CAD build for the part. Positions are in the model's coordinates, mm. A direction names the side the tool comes from. Give positions to 0.01 mm unless a question says otherwise; leave off trailing zeros. Loops run counter-clockwise (first coordinate to the right, second up) from the corner with the lowest first, then second, coordinate; pieces in that order, holes last. Notation, with made-up numbers: (-39, -13) -> (-33, -13) arc R25 ccw to (-33, 26) -> close; hole circle Ø4 at (-10, 28.5). An arc over 180 degrees is marked (long way). Write each question's results on one line, items separated by ' | '. Start each with the question number.
```python
from build123d import *

# Parameters (mm, degrees)
ESTRUSIONE_ESTRUSIONE1_DEPTH = 12.54
SCHIZZO3_R                   = 6.5
ESTRUSIONE_ESTRUSIONE2_DEPTH = 2.62
SCHIZZO4_R                   = 3
TAGLIO_ESTRUSIONE1_DEPTH     = 36.652428389
FORO_FILETTATO_M2_5X0_45_1_D = 2.05


with BuildPart() as part:
    # Schizzo1 → Rivoluzione1 (revolve)
    with BuildSketch(Plane.XY, mode=Mode.PRIVATE) as rivoluzione1_sk:
        with BuildLine():
            Line((0, 0), (9.485, 0))
            Line((9.485, 0), (9.485, -4.2))
            Line((9.485, -4.2), (14.505, -4.2))
            Line((14.505, -4.2), (14.505, -7.3))
            Line((14.505, -7.3), (10.745, -7.3))
            ThreePointArc((10.745, -7.3), (9.154009742, -7.959009742), (8.495, -9.55))
            Line((8.495, -9.55), (8.495, -14))
            Line((8.495, -14), (0, -14))
            Line((0, -14), (0, 0))
        make_face()
    revolve(rivoluzione1_sk.sketch.rotate(Axis((0, 0, 0), (0, -1, 0)), 180), axis=Axis((0, 0, 0), (0, -1, 0)))

    # Schizzo2 → Estrusione-Estrusione1 (add)
    with BuildSketch(Plane(origin=(0, 0, 0), x_dir=(1, 0, 0), z_dir=(0, 1, 0))):
        Polygon((2.090015263, -8.937889289), (3.249793028, -8.584455371), (8.785446812, -2.658938333), (9.059252943, -1.477824366), (6.695431549, 6.278950956), (5.809459915, 7.106631005), (-2.090015263, 8.937889289), (-3.249793028, 8.584455371), (-8.785446812, 2.658938333), (-9.059252943, 1.477824366), (-6.695431549, -6.278950956), (-5.809459915, -7.106631005), align=None)
    extrude(amount=ESTRUSIONE_ESTRUSIONE1_DEPTH)

    # Schizzo3 → Estrusione-Estrusione2 (add)
    with BuildSketch(Plane(origin=(0, 12.54, 0), x_dir=(1, 0, 0), z_dir=(0, 1, 0))):
        with Locations(Location((0, 0, 0), (0, 0, 180))):
            Circle(SCHIZZO3_R)
    extrude(amount=ESTRUSIONE_ESTRUSIONE2_DEPTH)

    # Schizzo4 → Taglio-Estrusione1 (cut, through all)
    with BuildSketch(Plane(origin=(0, 15.16, 0), x_dir=(1, 0, 0), z_dir=(0, 1, 0))):
        with Locations(Location((0, 0, 0), (0, 0, 180))):
            Circle(SCHIZZO4_R)
    extrude(amount=-TAGLIO_ESTRUSIONE1_DEPTH, mode=Mode.SUBTRACT)

    # Foro filettato M2.5x0.45-1 (through all)
    with Locations(Plane(origin=(0, -4.2, 0), x_dir=(1, 0, 0), z_dir=(0, 1, 0))):
        with Locations((0, -12), (-10.392304845, -6), (-10.392304845, 6), (0, 12), (10.392304845, 6), (10.392304845, -6), (0, 0)):
            Hole(FORO_FILETTATO_M2_5X0_45_1_D / 2)


solid = part.part
```
Q1. Saw through at C-C, the plane z = 0. List the corners of the cut face in (x, y) (3 decimals), then the cut area to 3 significant figures.
Q2. Which spindle directions (+Z, -Z, +X, -X, +Y, -Y) get a long thin tool onto all of the face, cutting with end or side? Do faces 1 (the face through (-6.259, 6.182, 6.687)), 2 (the face through (-8.92, 6.18, -2.08)), 3 (the face through (1.842, -11.806, 8.293)), 4 (the face through (5.158, 13.832, -3.955)), 5 (the face through (1.92, 6.18, -8.01)). Say none if no direction does.
Q3. Wall check: L1, parallel to X at y = -5.1, z = 6; L2, parallel to X at y = -0.75, z = -0.25; L3, parallel to Y at x = 8.5, z = -11.5. Give the ranges that are in metal, low to high.
Q4. Drop flat-ended pins along their axis: pin 1 (2.5 mm diameter, centred on x = -10.39, z = 6, fed in from -Y); pin 2 (2.5 mm diameter, centred on x = -10.39, z = -6, fed in from +Y); pin 3 (1.8 mm diameter, centred on x = 0, z = -12, fed in from -Y); pin 4 (1.5 mm diameter, centred on y = 11, z = 2.5, fed in from -X). Give the stop position or say it passes through.
Q5. Saw through at B-B, the plane y = -4.75. List the corners of the cut face in (x, z) (3 decimals), then the cut area to 3 significant figures.
Q6. Saw through at D-D, the plane x = 0. Give the number of separate pieces and of enclosed holes in the cut face, then the cut area to 3 significant figures.
Q7. Mould opens along X. For faces 6 (the face through (3.14, -5.77, 14.16)), 7 (the face through (0, 12.54, 7)), 8 (the face through (0.76, -5.77, 11.31)), 9 (the face through (8.92, 6.18, 2.08)) say: pulls with the +X half, pulls with the -X half, needs draft (parallel to the pull), parting line crosses it, or undercut.
Q8. Saw through at A-A, the plane y = 8.5. List the corners of the cut face in (x, z), then the cut area to 3 significant figures.
Answer block:
1) outline: (-14.505, -7.3) -> (-10.745, -7.3) arc R2.25 cw to (-8.495, -9.55) -> (-8.495, -14) -> (-3, -14) -> (-3, 15.16) -> (-6.5, 15.16) -> (-6.5, 12.54) -> (-8.609, 12.54) -> (-8.609, 0) -> (-9.485, 0) -> (-9.485, -4.2) -> (-14.505, -4.2) -> close; (3, -14) -> (8.495, -14) -> (8.495, -9.55) arc R2.25 cw to (10.745, -7.3) -> (14.505, -7.3) -> (14.505, -4.2) -> (9.485, -4.2) -> (9.485, 0) -> (8.609, 0) -> (8.609, 12.54) -> (6.5, 12.54) -> (6.5, 15.16) -> (3, 15.16) -> close | area: 361 mm2
2) face 1: +Z, -X, +Y | face 2: -Z, -X, +Y | face 3: -Y | face 4: +Y | face 5: -Z, +X, +Y
3) L1: x = -13.21 to -11.42, -9.37 to 9.37, 11.42 to 13.21 | L2: x = -9.48 to -2.99, 2.99 to 9.48 | L3: y = -7.3 to -4.2
4) pin 1: stops at y = -7.3 | pin 2: stops at y = -4.2 | pin 3: passes through | pin 4: stops at x = -8.08
5) outline: circle Ø29.01 at (0, 0); hole circle Ø2.05 at (-10.392, -6); hole circle Ø2.05 at (-10.392, 6); hole circle Ø6 at (0, 0); hole circle Ø2.05 at (0, -12); hole circle Ø2.05 at (0, 12); hole circle Ø2.05 at (10.392, -6); hole circle Ø2.05 at (10.392, 6) | area: 613 mm2
6) separate pieces: 4 | enclosed holes: 0 | area: 344 mm2
7) face 6: parting line crosses it | face 7: needs draft | face 8: undercut | face 9: pulls with the +X half
8) outline: (-9.06, -1.48) -> (-8.79, -2.66) -> (-3.25, -8.58) -> (-2.09, -8.94) -> (5.81, -7.11) -> (6.7, -6.28) -> (9.06, 1.48) -> (8.79, 2.66) -> (3.25, 8.58) -> (2.09, 8.94) -> (-5.81, 7.11) -> (-6.7, 6.28) -> close; hole circle Ø6 at (0, 0) | area: 205 mm2
